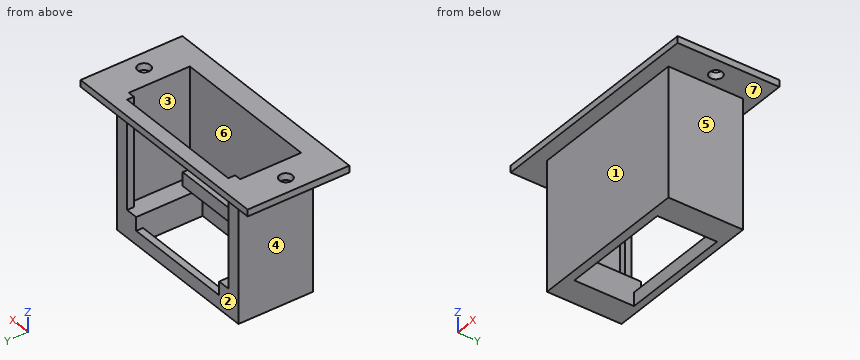
Autodesk Inventor part; units mm, degrees
ref_plane "YZ Plane" through (0, 0, 0) normal (1, 0, 0) x (0, 1, 0)
ref_plane "XZ Plane" through (0, 0, 0) normal (0, 1, 0) x (-1, 0, 0)
ref_plane "XY Plane" through (0, 0, 0) normal (0, 0, 1) x (1, 0, 0)
sketch "Sketch1" plane through (0, 0, 0) normal (0, 0, 1) x (1, 0, 0)
  line L0 (0, 0) -> (-41.91, 0)
  line L1 (-41.91, 0) -> (-41.91, 19.05)
  line L2 (-41.91, 19.05) -> (0, 19.05)
  line L3 (0, 19.05) -> (0, 0)
  circle A0 centre (-38.735, 9.525) radius 1.1938
  circle A1 centre (-3.175, 9.525) radius 1.1938
  dimension "d0" = 41.91
  dimension "d1" = 19.05
  dimension "d2" = 2.3876
  dimension "d3" = 2.3876
  dimension "d4" = 3.175
  dimension "d5" = 3.175
  dimension "d6" = 9.525
  dimension "d7" = 9.525
extrude "Extrusion1" add sketch "Sketch1" against normal blind 1.27
sketch "Sketch2" plane through (0, 0, 0) normal (0, 0, 1) x (1, 0, 0)
  line L0 (-41.91, 19.05) -> (-41.91, 0)
  line L1 (-36.195, 16.51) -> (-5.715, 16.51)
  line L2 (-5.715, 16.51) -> (-5.715, 2.54)
  line L3 (-5.715, 2.54) -> (-36.195, 2.54)
  line L4 (-36.195, 2.54) -> (-36.195, 16.51)
  line L5 (-41.91, 0) -> (0, 0)
  line L6 (0, 0) -> (0, 19.05)
  dimension "d31" = 13.97
  dimension "d32" = 2.54
  dimension "d33" = 30.48
  dimension "d34" = 5.715
extrude "Extrusion2" add sketch "Sketch2" against normal blind 25.4
sketch "Sketch3" plane through (0, 0, -25.4) normal (0, 0, -1) x (-1, 0, 0)
  line L0 (6.985, 15.24) -> (34.925, 15.24)
  line L1 (34.925, 15.24) -> (34.925, 3.81)
  line L2 (34.925, 3.81) -> (6.985, 3.81)
  line L3 (6.985, 3.81) -> (6.985, 15.24)
  line L4 (5.715, 16.51) -> (5.715, 2.54)
  line L5 (36.195, 16.51) -> (5.715, 16.51)
  line L6 (36.195, 2.54) -> (36.195, 16.51)
  line L7 (5.715, 2.54) -> (36.195, 2.54)
  point P0 (0, 0)
  dimension "d35" = 1.27
  dimension "d36" = 1.27
  dimension "d37" = 1.27
  dimension "d38" = 1.27
extrude "Extrusion3" cut sketch "Sketch3" against normal blind 25.4 contours L0 L1 L2 L3
sketch "Sketch4" plane through (0, 0, 0) normal (0, 0, 1) x (1, 0, 0)
  line L0 (-34.925, 15.24) -> (-6.985, 15.24)
  line L1 (-36.195, 16.51) -> (-5.715, 16.51)
  line L2 (-33.655, 15.24) -> (-8.255, 15.24)
  line L3 (-8.255, 15.24) -> (-8.255, 16.51)
  line L4 (-8.255, 16.51) -> (-33.655, 16.51)
  line L5 (-33.655, 16.51) -> (-33.655, 15.24)
  line L6 (-34.925, 3.81) -> (-34.925, 15.24)
  line L7 (-6.985, 15.24) -> (-6.985, 3.81)
  dimension "d39" = 1.27
  dimension "d40" = 1.27
extrude "Extrusion4" cut sketch "Sketch4" against normal blind 22.86
sketch "Sketch7" plane through (-34.925, 3.81, -25.4) normal (0, 1, 0) x (1, 0, 0)
  line L0 (0, 0) -> (0, -25.4)
  line L1 (26.67, -5.08) -> (0, -5.08)
  line L2 (0, -5.08) -> (0, -7.62)
  line L3 (0, -7.62) -> (26.67, -7.62)
  line L4 (26.67, -7.62) -> (26.67, -5.08)
  line L5 (0, 0) -> (27.94, 0)
  line L6 (26.67, -2.54) -> (26.67, -24.13)
  point P0 (34.925, -25.4)
  point P1 (0, -5.08)
  dimension "d54" = 2.54
  dimension "d55" = 5.08
extrude "Extrusion6" add sketch "Sketch7" along normal blind 2.286
sketch "Sketch8" plane through (-34.925, 3.81, -25.4) normal (0, 1, 0) x (1, 0, 0)
  line L0 (28.0721, -5.08) -> (24.384, -5.08)
  line L1 (24.384, -5.08) -> (24.384, 0)
  line L2 (24.384, 0) -> (27.94, 0)
  line L3 (0, -5.08) -> (3.556, -5.08)
  line L4 (3.556, -5.08) -> (3.556, 0)
  line L5 (3.556, 0) -> (0, 0)
  line L6 (0, 0) -> (0, -5.08)
  line L7 (0, 0) -> (27.94, 0)
  line L8 (27.94, 0) -> (27.94, -25.4)
  line L9 (27.94, -5.08) -> (27.94, 0)
  point P0 (34.925, -25.4)
  dimension "d46" = 3.556
  dimension "d47" = 5.08
  dimension "d48" = 3.556
  dimension "d49" = 5.08
extrude "Extrusion7" add sketch "Sketch8" along normal blind 12.7
sketch "Sketch9" plane through (-31.369, 3.81, -25.4) normal (0, 1, 0) x (1, 0, 0)
  line L0 (0, -5.08) -> (23.114, -5.08)
  line L1 (0, 0) -> (20.828, 0)
  line L2 (20.828, -5.08) -> (20.828, 0)
  line L3 (20.828, 0) -> (0, 0)
  line L4 (0, 0) -> (0, -5.08)
  line L5 (20.828, -5.08) -> (20.828, 0)
  line L6 (0, 0) -> (0, -5.08)
  line L7 (20.828, -5.08) -> (0, -5.08)
  point P0 (31.369, -25.4)
  point P1 (20.828, -5.08)
  point P2 (-3.556, 0)
  point P3 (-3.556, -5.08)
  point P4 (24.384, 0)
extrude "Extrusion8" add sketch "Sketch9" along normal blind 0.254
equation "\"d3\" = d2"
equation "\"d5\" = d4"
equation "\"d6\" = 0.5 * d1"
equation "\"d7\" = d6"
equation "\"d36\" = d35"
equation "\"d37\" = d35"
equation "\"d38\" = d36"
equation "\"d49\" = d47"
properties part number "_3DPrint"
Read the model definition and answer for the solid it produces. Units are mm, in the model's axes. Face numbers are marked on the shaded views. A direction names the side the tool comes from. Coordinates: 2 decimals unless noted, no trailing zeros. Write each loop counter-clockwise with the first axis right and the second up, starting at its lowest first coordinate (ties: lowest second). Pieces come first, ordered by that corner, then holes. Notation, with made-up numbers: (-7.75, 70) - (8.25, 70) arc R7 ccw to (8.25, 81) - close; hole circle Ø9 at (-0.75, -31.75). An arc over 180 degrees is marked (long way). One line per question, with ' | ' between items.
Q1. For the marked faces 1, 2, 3 and 4, determine the directions among +Z, -Z, +X, -X, +Y, -Y from which every point of the face is accessible in a straight line to the end or side of a thin tool.
Result set:
face 1: -Z, +X, -X, -Y | face 2: -Z, +X, -X, +Y | face 3: +Z | face 4: -Z, -X, +Y, -Y
Q2. Find section C-C, the plane y = 13.75. Write down the section's boundary in (x, z) (3 decimals).
Result set:
outline: (-41.91, -1.27) - (-36.195, -1.27) - (-36.195, -25.4) - (-31.369, -25.4) - (-31.369, -20.32) - (-34.925, -20.32) - (-34.925, 0) - (-41.91, 0) - close; (-10.541, -25.4) - (-5.715, -25.4) - (-5.715, -1.27) - (0, -1.27) - (0, 0) - (-6.985, 0) - (-6.985, -20.32) - (-10.541, -20.32) - close
Q3. Each of these flat-tipped pins is pushed along its axis until it touches: P1, Ø4, axis at x = -3.175, y = 9.525, coming from the -Z side; P2, Ø3.5, axis at y = 9.5, z = -6.5, coming from the +X side (3 decimals); P3, Ø3, axis at x = -21.5, z = -19, coming from the +Y side. Where does it stop, or does it pass through?
Result set:
P1: z = -1.27 | P2: x = -5.715 | P3: y = 6.1
Q4. Determine the mould class of the marked faces 5, 6 and 7 for opening direction X: +X half, -X half, draft (parallel to the pull), parting line (faces both ways), or undercut.
Result set:
face 5: +X half | face 6: undercut | face 7: draft
Q5. Find section A-A, the plane z = -23.5. Write down the section's boundary in (x, y) (3 decimals).
Result set:
outline: (-36.195, 2.54) - (-5.715, 2.54) - (-5.715, 16.51) - (-36.195, 16.51) - close; hole (-31.369, 4.064) - (-10.541, 4.064) - (-10.541, 15.24) - (-31.369, 15.24) - close
Q6. Consider L1, parallel to X at y = 9.25, z = -21.5 (3 decimals); L2, parallel to X at y = 5, z = -15.75 (3 decimals); L3, parallel to Y at x = -26, z = -11.75. Determine where each line is inside the solid, lowest interval first. Write a range as [from, to].
Result set:
L1: [-36.195, -31.369], [-10.541, -5.715] | L2: [-36.195, -34.925], [-6.985, -5.715] | L3: [2.54, 3.81]
Q7. Find section D-D, the plane x = -38.5. Write down the section's boundary in (y, z).
Result set:
outline: (0, -1.27) - (8.35, -1.27) - (8.35, 0) - (0, 0) - close; (10.7, -1.27) - (19.05, -1.27) - (19.05, 0) - (10.7, 0) - close
Q8. Find section B-B, the plane x = -19. Write down the section's boundary in (y, z), plus the area to 3 significant figures.
Result set:
outline: (0, -1.27) - (2.54, -1.27) - (2.54, -25.4) - (4.06, -25.4) - (4.06, -20.32) - (6.1, -20.32) - (6.1, -17.78) - (3.81, -17.78) - (3.81, 0) - (0, 0) - close; (15.24, -25.4) - (16.51, -25.4) - (16.51, -22.86) - (15.24, -22.86) - close; (16.51, -1.27) - (19.05, -1.27) - (19.05, 0) - (16.51, 0) - close | area: 49.0 mm^2
